Part model, mm, in its own coordinate system. A direction names the side the tool comes from. Give positions to 0.01 mm unless a question says otherwise; leave off trailing zeros. Order: outer loops, then holes, each group sorted by start corner. A loop starts at its lowest first (then second) coordinate and runs counter-clockwise, first axis right, second up. Notation, with made-up numbers: (-23, 7) - (8, 7) arc R18 ccw to (8, 22) - close; hole circle Ø2 at (76.25, 62.25). An arc over 180 degrees is marked (long way). One line per item, written item: value.
```python
from build123d import *

# Parameters (mm, degrees)
SKETCH1_W           = 3.175
SKETCH1_H           = 13
SKETCH1_H_2         = 5
BOSS_EXTRUDE1_DEPTH = 3.175
FILLET2_R           = 3
FILLET3_R           = 3


with BuildPart() as part:
    # Sketch1 → Boss-Extrude1 (new body)
    with BuildSketch(Plane.XY):
        Polygon((-80, -25), (-76.2, -25), (76.2, -25), (80, -25), (80, 25), (-80, 25), (-80, 8), (-80, 3), (-80, -7), align=None)
        with Locations((-74.6125, -13.5)):
            Rectangle(SKETCH1_W, SKETCH1_H, mode=Mode.SUBTRACT)
        with Locations((74.6125, -13.5)):
            Rectangle(SKETCH1_W, SKETCH1_H, mode=Mode.SUBTRACT)
        with Locations((-74.6125, 5.5)):
            Rectangle(SKETCH1_W, SKETCH1_H_2, mode=Mode.SUBTRACT)
        with Locations((74.6125, 5.5)):
            Rectangle(SKETCH1_W, SKETCH1_H_2, mode=Mode.SUBTRACT)
    extrude(amount=BOSS_EXTRUDE1_DEPTH)

    # Fillet2
    fillet2_edges = [part.edges().sort_by_distance(p)[0] for p in [
        (-80, 25, 1.5875),
    ]]
    fillet(fillet2_edges, radius=FILLET2_R)

    # Fillet3
    fillet3_edges = [part.edges().sort_by_distance(p)[0] for p in [
        (80, -25, 1.5875),
        (-80, -25, 1.5875),
        (80, 25, 1.5875),
    ]]
    fillet(fillet3_edges, radius=FILLET3_R)


solid = part.part
```
1) Wall check: line 1 along X through (y, z) = (-18, 2.6) (3 decimals). Give the ranges that are in metal, low to high. Write a range as [from, to].
Answer:
line 1: x = [-80, -76.2], [-73.025, 73.025], [76.2, 80]
2) Which spindle directions (+Z, -Z, +X, -X, +Y, -Y) get a long thin tool onto all of the face, cutting with end or side? Do faces 1 (the face through (-1, -25, 2)), 2 (the face through (-75, 3, 2)). Say none if no direction does.
Answer:
face 1: +Z, -Z, +X, -X, -Y
face 2: +Z, -Z
3) Slice it at A-A on y = -10.5. Write the cut outline in (x, z) (3 decimals), then the cut area to 3 significant figures.
Answer:
outline: (-80, 0) - (-76.2, 0) - (-76.2, 3.175) - (-80, 3.175) - close; (-73.025, 0) - (73.025, 0) - (73.025, 3.175) - (-73.025, 3.175) - close; (76.2, 0) - (80, 0) - (80, 3.175) - (76.2, 3.175) - close
area: 488 mm2
4) Two-plate mould, pull along X, no slides. Class faces 3 (the face through (79.1, -24.14, 1.61)), 4 (the face through (75, -7, 2)), 5 (the face through (-79.14, -24.1, 1.61)): pulls with the +X half, pulls with the -X half, needs draft (parallel to the pull), parting line crosses it, or undercut.
Answer:
face 3: pulls with the +X half
face 4: undercut
face 5: pulls with the -X half
5) Slice it at B-B on z = 2.2. Write the cut outline in (x, y) (3 decimals).
Answer:
outline: (-80, -22) arc R3 ccw to (-77, -25) - (77, -25) arc R3 ccw to (80, -22) - (80, 22) arc R3 ccw to (77, 25) - (-77, 25) arc R3 ccw to (-80, 22) - close; hole (-76.2, -20) - (-73.025, -20) - (-73.025, -7) - (-76.2, -7) - close; hole (-76.2, 3) - (-73.025, 3) - (-73.025, 8) - (-76.2, 8) - close; hole (73.025, -20) - (76.2, -20) - (76.2, -7) - (73.025, -7) - close; hole (73.025, 3) - (76.2, 3) - (76.2, 8) - (73.025, 8) - close
